Source: CAD feature listing. Evaluate the final solid. Frame: model axes, mm. Face numbers are marked on the shaded views. Coordinates: 2 decimals unless noted, no trailing zeros. Write each loop counter-clockwise with the first axis right and the second up, starting at its lowest first coordinate (ties: lowest second). Pieces come first, ordered by that corner, then holes. Notation, with made-up numbers: M 62,3 L 88,3 A33 ccw 88,41 Z; hole C -8.75,75.25 d6. An arc over 180 degrees is marked long. Answer as CSV lines item,"result". Start each with the question number.
1. Mould query, pull axis Y, two halves, no side actions, for the marked faces 1, 2 and 3. Classes: pulls with the +Y half, pulls with the -Y half, needs draft (parallel to the pull), parting line crosses it, or undercut.
2. Section C-C on x = 0. Return the cut outline in (y, z), plus the area to 3 significant figures.
3. Line query: probe 1 along X at (y, z) = (0, 0.5); probe 2 along Y at (x, z) = (0, 0); probe 3 along X at (y, z) = (-1.75, 2.75). Output: solid intervals per line, ascending. Write a range as [from, to].
4. Section B-B on z = -1. Return the cut outline in (x, y).
5. Section A-A on y = 0. Return the cut outline in (x, z), plus the area to 3 significant figures.
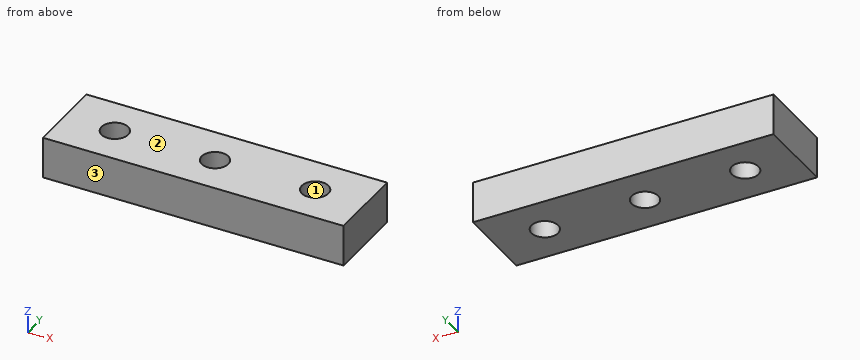
Solid Edge part; units mm, degrees
sketch "Sketch1" plane through (0, 0, 0) normal (0, 0, 1) x (1, 0, 0)
  line L0 (-22.5, -6) -> (22.5, -6)
  line L1 (22.5, -6) -> (22.5, 6)
  line L2 (22.5, 6) -> (-22.5, 6)
  line L3 (-22.5, 6) -> (-22.5, -6)
  dimension "D1" = 22.5
  dimension "D2" = 22.5
extrude "Protrusion1" add sketch "Sketch1" along normal mid plane 6.2
hole "Hole_1" at (-15, 0, 3.1) direction (0, 0, -1) diameter 4 end up to next
hole "Hole1" at (0, 0, 3.1) direction (0, 0, -1) diameter 4 end up to next
hole "Hole2" at (15, 0, 3.1) direction (0, 0, -1) diameter 4 end up to next
properties material "Polyethylene, low density"
Values:
1,face 1,"undercut"
1,face 2,"needs draft"
1,face 3,"pulls with the -Y half"
2,outline,"M -6,-3.1 L -2,-3.1 L -2,3.1 L -6,3.1 Z; M 2,-3.1 L 6,-3.1 L 6,3.1 L 2,3.1 Z"
2,area,"49.6 mm²"
3,probe 1,"[-22.5, -17], [-13, -2], [2, 13], [17, 22.5]"
3,probe 2,"[-6, -2], [2, 6]"
3,probe 3,"[-22.5, -15.97], [-14.03, -0.97], [0.97, 14.03], [15.97, 22.5]"
4,outline,"M -22.5,-6 L 22.5,-6 L 22.5,6 L -22.5,6 Z; hole C -15,0 d4; hole C 0,0 d4; hole C 15,0 d4"
5,outline,"M -22.5,-3.1 L -17,-3.1 L -17,3.1 L -22.5,3.1 Z; M -13,-3.1 L -2,-3.1 L -2,3.1 L -13,3.1 Z; M 2,-3.1 L 13,-3.1 L 13,3.1 L 2,3.1 Z; M 17,-3.1 L 22.5,-3.1 L 22.5,3.1 L 17,3.1 Z"
5,area,"205 mm²"
